Input: part model. Units: mm. Frame: model coordinates. A direction names the side the tool comes from. Coordinates: 2 decimals unless noted, no trailing zeros. Order: outer loops, then holes, each group sorted by start corner. A loop starts at its lowest first (then second) coordinate and runs counter-clockwise, first axis right, second up. Notation, with made-up numbers: (15, 33.25) -> (67, 33.25) arc R6 ccw to (67, 38.25) -> close; hole circle Ø3 at (5.5, 72). An arc over 180 degrees is marked (long way). One line per question, with ' | ' between items.
```python
from build123d import *

# Parameters (mm, degrees)
EXTRUDE_1_DEPTH          = 7
CUT_EXTRUDE_1_DEPTH      = 34.339166156
CUT_EXTRUDE_1_DEPTH_BACK = 34.339166156
SKETCH_2_R               = 2.1
FILLET_1_R               = 4
CUT_EXTRUDE_2_DEPTH      = 26.689773137
CUT_EXTRUDE_2_DEPTH_BACK = 26.689773137
SKETCH_3_R               = 2


with BuildPart() as part:
    # Эскиз1 → Бобышка-Вытянуть1 (new body)
    with BuildSketch(Plane(origin=(0, 0, 0), x_dir=(1, 0, 0), z_dir=(0, 1, 0))):
        with BuildLine():
            Line((0, 10.75), (0, 12.25))
            Line((0, 12.25), (-10.3, 12.25))
            ThreePointArc((-10.3, 12.25), (-18.219595949, 8.969595949), (-21.5, 1.05))
            Line((-21.5, 1.05), (-21.5, -1.05))
            ThreePointArc((-21.5, -1.05), (-18.219595949, -8.969595949), (-10.3, -12.25))
            Line((-10.3, -12.25), (0, -12.25))
            Line((0, -12.25), (0, -10.75))
            Line((0, -10.75), (-11, -10.75))
            ThreePointArc((-11, -10.75), (-17.363961031, -8.113961031), (-20, -1.75))
            Line((-20, -1.75), (-20, 1.75))
            ThreePointArc((-20, 1.75), (-17.363961031, 8.113961031), (-11, 10.75))
            Line((-11, 10.75), (0, 10.75))
        make_face()
    extrude(amount=EXTRUDE_1_DEPTH)

    # Эскиз2 → Вырез-Вытянуть1 (cut, two sides: drawn at the far end of the back side and taken through both)
    with BuildSketch(Plane.XY.offset(12.25).offset(-CUT_EXTRUDE_1_DEPTH_BACK)):
        with Locations((-3.5, 3.5)):
            Circle(SKETCH_2_R)
    extrude(amount=CUT_EXTRUDE_1_DEPTH + CUT_EXTRUDE_1_DEPTH_BACK, mode=Mode.SUBTRACT)

    # Скругление1
    # the kernel refuses this fillet: 4 mm, written as the material it takes off along each edge
    with BuildSketch(Plane(origin=(0, 0, -0.75), x_dir=(-1, 0, 0), z_dir=(0, 0, -1)), Plane(origin=(0, 0, 22.25), x_dir=(-1, 0, 0), z_dir=(0, 0, -1))) as fillet_1_piece_1:
        with BuildLine():
            CenterArc((FILLET_1_R, FILLET_1_R), FILLET_1_R, 180, 90)
            Line((0, FILLET_1_R), (0, 0))
            Line((0, 0), (FILLET_1_R, 0))
        make_face()
    extrude(amount=21.5, mode=Mode.SUBTRACT)
    with BuildSketch(Plane(origin=(0, 7, -0.75), x_dir=(-1, 0, 0), z_dir=(0, 0, -1)), Plane(origin=(0, 7, 22.25), x_dir=(-1, 0, 0), z_dir=(0, 0, -1))) as fillet_1_piece_2:
        with BuildLine():
            CenterArc((FILLET_1_R, -FILLET_1_R), FILLET_1_R, 90, 90)
            Line((0, -FILLET_1_R), (0, 0))
            Line((0, 0), (FILLET_1_R, 0))
        make_face()
    extrude(amount=21.5, mode=Mode.SUBTRACT)

    # Эскиз3 → Вырез-Вытянуть2 (cut, two sides: drawn at the far end of the back side and taken through both)
    with BuildSketch(Plane.ZY.offset(21.5).offset(-CUT_EXTRUDE_2_DEPTH_BACK)):
        with Locations(Location((0, 3.5, 0), (0, 0, 28.955024372))):
            Circle(SKETCH_3_R)
    extrude(amount=CUT_EXTRUDE_2_DEPTH + CUT_EXTRUDE_2_DEPTH_BACK, mode=Mode.SUBTRACT)


solid = part.part
```
1. Access query for faces 1 (the face through (-21.5, 6, 0)), 2 (the face through (-7, 3, -10.75)). Directions: +Z, -Z, +X, -X, +Y, -Y. A direction counts if a zero-diameter tool reaches every point of the face in a straight line with its end or side. Return the directions, or none.
Recorded:
face 1: +Z, -Z, -X, +Y, -Y | face 2: +X, +Y, -Y
2. Ray query, line 1 (Z direction, x = -2, y = 1.25); line 2 (Y direction, x = -20.5, z = 0); line 3 (Z direction, x = -18, y = 1.25). Return the intervals inside material, ascending. Write a range as [from, to].
Recorded:
line 1: z = [-12.25, -10.75], [10.75, 12.25] | line 2: y = [0, 1.5], [5.5, 7] | line 3: z = [-9.18, -7.41], [7.41, 9.18]
3. Mould query, pull axis Y, two halves, no side actions, for faces 3 (the face through (-20, 1, 0)), 4 (the face through (-1.32, 1.03, -11.49)), 5 (the face through (-3.96, 1.45, -11.51)). Classes: released by +Y, released by -Y, zero draft, split by the parting line, or undercut.
Recorded:
face 3: zero draft | face 4: released by -Y | face 5: undercut
4. Cut plane D-D, the plane y = 3. Return loops of the section in (x, z).
Recorded:
outline: (-21.46, -1.94) arc R11.2 ccw to (-10.3, -12.25) -> (-5.54, -12.25) -> (-5.54, -10.75) -> (-11, -10.75) arc R9 cw to (-20, -1.94) -> close; (-21.46, 1.94) -> (-20, 1.94) arc R9 cw to (-11, 10.75) -> (-5.54, 10.75) -> (-5.54, 12.25) -> (-10.3, 12.25) arc R11.2 ccw to start; (-1.46, -12.25) -> (-0.13, -12.25) -> (-0.13, -10.75) -> (-1.46, -10.75) -> close; (-1.46, 10.75) -> (-0.13, 10.75) -> (-0.13, 12.25) -> (-1.46, 12.25) -> close
5. Cut plane C-C, the plane x = -17.5. Return loops of the section in (y, z).
Recorded:
outline: (0, -9.63) -> (7, -9.63) -> (7, -7.97) -> (0, -7.97) -> close; (0, 7.97) -> (7, 7.97) -> (7, 9.63) -> (0, 9.63) -> close
6. Cut plane B-B, the plane x = -3. Return loops of the section in (y, z), and give its area (3 significant figures).
Recorded:
outline: (0.13, -12.25) -> (1.46, -12.25) -> (1.46, -10.75) -> (0.13, -10.75) -> close; (0.13, 10.75) -> (1.46, 10.75) -> (1.46, 12.25) -> (0.13, 12.25) -> close; (5.54, -12.25) -> (6.87, -12.25) -> (6.87, -10.75) -> (5.54, -10.75) -> close; (5.54, 10.75) -> (6.87, 10.75) -> (6.87, 12.25) -> (5.54, 12.25) -> close | area: 8.00 mm^2
7. Cut plane A-A, the plane z = 0. Return loops of the section in (x, y).
Recorded:
outline: (-21.5, 0) -> (-20, 0) -> (-20, 1.5) -> (-21.5, 1.5) -> close; (-21.5, 5.5) -> (-20, 5.5) -> (-20, 7) -> (-21.5, 7) -> close
8. Pin query (flat end, axial travel): pin 1 Ø0.8 at (y, z) = (5.5, 0) entering from +X; pin 2 Ø3 at (y, z) = (1.5, 3) entering from +X; pin 3 Ø3 at (x, y) = (-15.5, 2) entering from +Z. Return the tip coordinate at first contact, or that it passes through.
Recorded:
pin 1: stops at x = -20 | pin 2: stops at x = -19.57 | pin 3: stops at z = 11.62
